from build123d import *

# Parameters (mm, degrees)
BOSS_EXTRUDE1_DEPTH = 8
FILLET1_R           = 25


with BuildPart() as part:
    # Sketch1 → Boss-Extrude1 (new body)
    with BuildSketch(Plane.XY):
        with BuildLine():
            Line((0, 0), (15, 0))
            Line((15, 0), (23.956669948, 12.610236454))
            ThreePointArc((23.956669948, 12.610236454), (22.027601971, 16.399841272), (20.011882934, 12.655607746))
            Line((20.011882934, 12.655607746), (20.674588623, 13.103738497))
            ThreePointArc((20.674588623, 13.103738497), (22.018401314, 15.599894181), (23.304446632, 13.07349097))
            Line((23.304446632, 13.07349097), (14.586956827, 0.8))
            Line((14.586956827, 0.8), (0, 0.8))
            Line((0, 0.8), (0, 0))
        make_face()
    extrude(amount=BOSS_EXTRUDE1_DEPTH)

    # Fillet1
    fillet1_edges = [part.edges().sort_by_distance(p)[0] for p in [
        (14.586956827, 0.8, 4),
        (15, 0, 4),
    ]]
    fillet(fillet1_edges, radius=FILLET1_R)


solid = part.part
Geometry check sheet. Reference: the model listing, model coordinates, mm. A direction names the side the tool comes from. Round coordinates to 2 decimals unless told otherwise and drop trailing zeros. Order: outer loops, then holes, each group sorted by start corner. A loop starts at its lowest first (then second) coordinate and runs counter-clockwise, first axis right, second up. Notation, with made-up numbers: M 80,81 L 116,81 A25 ccw 116,107 Z; hole C 44.25,29 d2. An arc over 180 degrees is marked long. Answer in a Markdown table with one row per item.
(1) Sectioned sample at C-C, the plane x = 15.5. Record the cut outline in (y, z), and give its area (3 significant figures).
Responses:
| item | result |
|---|---|
| outline | M 3.9,0 L 4.97,0 L 4.97,8 L 3.9,8 Z |
| area | 8.55 mm² |
(2) Sectioned sample at D-D, the plane y = 4.5. Record the cut outline in (x, z).
Responses:
| item | result |
|---|---|
| outline | M 14.77,0 L 16.4,0 L 16.4,8 L 14.77,8 Z |
(3) Tool access check on faces 1 (the face through (1, 0, 4)), 2 (the face through (22.69, 12.21, 3.94)), 3 (the face through (13.296, 3.663, 4.056)). Record the directions out of +Z, -Z, +X, -X, +Y, -Y that give a thin tool (end or side, any length) a straight path to the whole face; none if there is none.
Responses:
| item | result |
|---|---|
| face 1 | +Z, -Z, +X, -X, -Y |
| face 2 | +Z, -Z |
| face 3 | +Z, -Z, -X |
(4) Scan lines: probe 1 along X at (y, z) = (14, 5.75); probe 2 along Y at (x, z) = (22.75, 7.5); probe 3 along Y at (x, z) = (22, 2.5). Record each from-to range of solid material in increasing order. Write a range as from..to.
Responses:
| item | result |
|---|---|
| probe 1 | x = 19.6..20.4, 23.6..24.4 |
| probe 2 | y = 10.91..12.29, 15.41..16.28 |
| probe 3 | y = 9.88..11.24, 15.6..16.4 |
(5) Sectioned sample at A-A, the plane y = 14. Record the cut outline in (x, z).
Responses:
| item | result |
|---|---|
| outline | M 19.6,0 L 20.4,0 L 20.4,8 L 19.6,8 Z; M 23.6,0 L 24.4,0 L 24.4,8 L 23.6,8 Z |
(6) Go/stop test with flat-tipped pins: P1, Ø1.5, axis at y = 11.5, z = 5, coming from the -X side; P2, Ø0.5, axis at x = 1, z = 5, coming from the +Y side; P3, Ø1, axis at y = 5.5, z = 6.5, coming from the -X side; P4, Ø3, axis at x = 22, y = 14, coming from the +Z side. Record where each tip stops, or that it passes through.
Responses:
| item | result |
|---|---|
| P1 | stops at x = 21.64 |
| P2 | stops at y = 0.8 |
| P3 | stops at x = 15.55 |
| P4 | passes through |
(7) Sectioned sample at B-B, the plane z = 2. Record the cut outline in (x, y), and give its area (3 significant figures).
Responses:
| item | result |
|---|---|
| outline | M 0,0 L 2.09,0 A25 ccw 22.47,10.52 L 23.96,12.61 A2.4 ccw long 20.01,12.66 L 20.67,13.1 A1.6 cw long 23.3,13.07 L 22.06,11.32 A25 cw 1.68,0.8 L 0,0.8 Z |
| area | 31.0 mm² |
(8) Draft check along Y on faces 4 (the face through (23.205, 11.552, 3.944)), 5 (the face through (22, 15.6, 3.9)), 6 (the face through (1, 0.8, 4)), 7 (the face through (18, 6, 8)). Enter one of: released by +Y, released by -Y, zero draft, split by the parting line, or undercut.
Responses:
| item | result |
|---|---|
| face 4 | released by -Y |
| face 5 | undercut |
| face 6 | released by +Y |
| face 7 | zero draft |
